Check sheet for the modelled part. Datum: model origin and axes. Units: mm. A direction names the side the tool comes from. Give positions to 0.01 mm unless a question says otherwise; leave off trailing zeros. Write each loop counter-clockwise with the first axis right and the second up, starting at its lowest first coordinate (ties: lowest second). Pieces come first, ordered by that corner, then holes. Notation, with made-up numbers: (68, 9.5) -> (124, 9.5) arc R3 ccw to (124, 13.5) -> close; hole circle Ø3 at (29, 33). An arc over 180 degrees is marked (long way). Use a Markdown table: item, result. Add a question column.
1. Cross-section at C-C (x = -41). Enter the section's corners in (y, z) (1 decimal).
2. Gauge pin test, flat ends, axial feed: P1, Ø1.5, axis at y = -63, z = 8, coming from the -X side; P2, Ø4, axis at x = -23.1, y = 0, coming from the +Z side; P3, Ø8, axis at x = 5.5, y = 16.5, coming from the +Z side. Record the tip position at first contact, or that the pin passes through.
3. Cross-section at A-A (x = 5). Enter the section's corners in (y, z) (1 decimal).
4. Release check for a two-part mould opening along Y. For faces 1 (the cylindrical face through (6.46, -73.07, 1.52)), 2 (the flat face through (5, -64, 3)) record: released by +Y, released by -Y, zero draft, split by the parting line, or undercut.
5. Set-up check for faces 3 (the flat face through (10, -64, 1)), 4 (the flat face through (-35, -53, 0)), 5 (the flat face through (-34, -75.359, 4)), 6 (the cylindrical face through (-12.005, -0.533, 6.535)), 7 (the flat face through (-65.048, -65, 8)): record each of +Z, -Z, +X, -X, +Y, -Y from which the full face is reachable in a straight line by a thin tool's end or side.
6. Cross-section at B-B (y = 0). Enter the section's corners in (x, z).
7. Scan lines: probe 1 along Y at (x, z) = (-33.5, 3) (3 decimals); probe 2 along Y at (x, z) = (5, 1.2) (3 decimals); probe 3 along Y at (x, z) = (-22.5, 8.5) (3 decimals). Record each from-to range of solid material in increasing order. Write a range as [from, to].
8. Cross-section at D-D (y = 30). Enter the section's corners in (x, z).
from build123d import *

# Parameters (mm, degrees)
PAD_DEPTH            = 83.675
POCKET001_DEPTH      = 5
SKETCH003_R          = 1.58
POCKET002_DEPTH      = 9.001
SKETCH006_R          = 1.58
POCKET_DEPTH         = 379.711606
POCKET_DEPTH_BACK    = 388.711606
SKETCH008_R          = 1.58
POCKET004_DEPTH      = 0.001
POCKET004_DEPTH_BACK = 9.001
POCKET005_DEPTH      = 0.001
POCKET005_DEPTH_BACK = 9.001
POCKET006_DEPTH      = 79.208699
POCKET006_DEPTH_BACK = 10.001
POCKET007_DEPTH      = 0.001
POCKET007_DEPTH_BACK = 9.001
POCKET008_DEPTH      = 3


with BuildPart() as part:
    # Sketch → Pad (new body, symmetric)
    with BuildSketch(Plane.XZ):
        Polygon((-6, 9), (-79.207699, 9), (-79.207699, 0), (0, 0), (10, 0), (10, 3), (0, 3), (0, 9), align=None)
    extrude(amount=PAD_DEPTH, both=True)

    # Sketch002 → Pocket001 (cut)
    with BuildSketch(Plane.XY.offset(9)):
        with BuildLine():
            Line((-34.353849, 27.1), (-39.603849, 27.1))
            Line((-39.603849, 27.1), (-44.853849, 27.1))
            ThreePointArc((-44.853849, 27.1), (-67.207699, 0), (-44.853849, -27.1))
            Line((-44.853849, -27.1), (-34.353849, -27.1))
            ThreePointArc((-34.353849, -27.1), (-12, 0), (-34.353849, 27.1))
        make_face()
    extrude(amount=-POCKET001_DEPTH, mode=Mode.SUBTRACT)

    # Sketch003 → Pocket002 (cut, through all)
    with BuildSketch(Plane.XY):
        with Locations((-50.806289, -19.403194)):
            Circle(SKETCH003_R)
        with Locations((-28.40141, -19.403194)):
            Circle(SKETCH003_R)
        with Locations((-28.40141, 19.403194)):
            Circle(SKETCH003_R)
        with Locations((-50.806289, 19.403194)):
            Circle(SKETCH003_R)
        with Locations((-62.008728, 0)):
            Circle(SKETCH003_R)
        with Locations((-56.108728, 0)):
            Circle(SKETCH003_R)
        with Locations((-17.198971, 0)):
            Circle(SKETCH003_R)
        with Locations((-23.098971, 0)):
            Circle(SKETCH003_R)
    extrude(amount=POCKET002_DEPTH, mode=Mode.SUBTRACT)

    # Sketch006 → Pocket (cut, two sides)
    with BuildSketch(Plane.XY) as pocket_sk:
        with Locations((5, 73.675)):
            Circle(SKETCH006_R)
    pocket = extrude(amount=-POCKET_DEPTH, mode=Mode.SUBTRACT) + extrude(pocket_sk.sketch, amount=POCKET_DEPTH_BACK, mode=Mode.SUBTRACT)

    # Mirrored: Pocket across Sketch006 H_Axis
    add(pocket.mirror(Plane.ZX), mode=Mode.SUBTRACT)

    # Sketch008 → Pocket004 (cut, two sides)
    with BuildSketch(Plane.XY) as pocket004_sk:
        with Locations((-70.627699, -68.515)):
            Circle(SKETCH008_R)
        with Locations((-70.627699, -60.515)):
            Circle(SKETCH008_R)
    extrude(amount=-POCKET004_DEPTH, mode=Mode.SUBTRACT)
    extrude(pocket004_sk.sketch, amount=POCKET004_DEPTH_BACK, mode=Mode.SUBTRACT)

    # Sketch005 → Pocket005 (cut, two sides)
    with BuildSketch(Plane.XY) as pocket005_sk:
        with BuildLine():
            ThreePointArc((-5.147488, 84.556872), (-51.101438, 66.874328), (-79.207699, 26.445674))
            Line((-79.207699, 26.445674), (-107.360429, 26.445674))
            Line((-107.360429, 26.445674), (-107.360429, 113.139377))
            Line((-5.147488, 113.139377), (-107.360429, 113.139377))
            Line((-5.147488, 84.556872), (-5.147488, 113.139377))
        make_face()
    extrude(amount=-POCKET005_DEPTH, mode=Mode.SUBTRACT)
    extrude(pocket005_sk.sketch, amount=POCKET005_DEPTH_BACK, mode=Mode.SUBTRACT)

    # Sketch009 → Pocket006 (cut, two sides)
    with BuildSketch(Plane.YZ) as pocket006_sk:
        with BuildLine():
            ThreePointArc((-33.515, 0), (-40.015, 4), (-46.515, 0))
            Line((-40.015, 0), (-46.515, 0))
            Line((-40.015, 0), (-33.515, 0))
        make_face()
    extrude(amount=-POCKET006_DEPTH, mode=Mode.SUBTRACT)
    extrude(pocket006_sk.sketch, amount=POCKET006_DEPTH_BACK, mode=Mode.SUBTRACT)

    # Sketch010 → Pocket007 (cut, two sides)
    with BuildSketch(Plane.XY) as pocket007_sk:
        with BuildLine():
            ThreePointArc((-44.458302, -55.549289), (-54.363008, -65.453995), (-44.458302, -75.358701))
            Line((-44.458302, -75.358701), (-22.419182, -75.358701))
            ThreePointArc((-22.419182, -75.358701), (-12.514476, -65.453995), (-22.419182, -55.549289))
            Line((-22.419182, -55.549289), (-44.458302, -55.549289))
        make_face()
    extrude(amount=-POCKET007_DEPTH, mode=Mode.SUBTRACT)
    extrude(pocket007_sk.sketch, amount=POCKET007_DEPTH_BACK, mode=Mode.SUBTRACT)

    # Sketch007 → Pocket008 (cut)
    with BuildSketch(Plane.XY.offset(9)):
        with BuildLine():
            Line((-79.207699, -64.515), (-79.207699, -68.515))
            Line((-76.207699, -68.515), (-79.207699, -68.515))
            ThreePointArc((-76.207699, -68.515), (-70.627699, -74.095), (-65.047699, -68.515))
            Line((-65.047699, -68.515), (-65.047699, -64.515))
            Line((-65.047699, -60.515), (-65.047699, -64.515))
            ThreePointArc((-65.047699, -60.515), (-70.627699, -54.935), (-76.207699, -60.515))
            Line((-76.207699, -60.515), (-79.207699, -60.515))
            Line((-79.207699, -64.515), (-79.207699, -60.515))
        make_face()
    extrude(amount=-POCKET008_DEPTH, mode=Mode.SUBTRACT)


solid = part.part
Worked answers:
| question | item | result |
|---|---|---|
| 1 | outline | (-83.7, 0) -> (-75.4, 0) -> (-75.4, 9) -> (-83.7, 9) -> close; (-55.5, 0) -> (-46.5, 0) arc R7.3 cw to (-33.5, 0) -> (73.7, 0) -> (73.7, 9) -> (27.1, 9) -> (27.1, 4) -> (-27.1, 4) -> (-27.1, 9) -> (-55.5, 9) -> close |
| 2 | P1 | stops at x = -65.05 |
| 2 | P2 | stops at z = 4 |
| 2 | P3 | stops at z = 3 |
| 3 | outline | (-83.7, 0) -> (-75.3, 0) -> (-75.3, 3) -> (-83.7, 3) -> close; (-72.1, 0) -> (-46.5, 0) arc R7.3 cw to (-43.7, 3) -> (-72.1, 3) -> close; (-36.3, 3) arc R7.3 cw to (-33.5, 0) -> (72.1, 0) -> (72.1, 3) -> close; (75.3, 0) -> (83.7, 0) -> (83.7, 3) -> (75.3, 3) -> close |
| 4 | face 1 | undercut |
| 4 | face 2 | zero draft |
| 5 | face 3 | +Z, -Z, +X, +Y, -Y |
| 5 | face 4 | -Z, +X, -X, +Y, -Y |
| 5 | face 5 | +Z, -Z |
| 5 | face 6 | +Z |
| 5 | face 7 | +Z, -X |
| 6 | outline | (-79.21, 0) -> (-63.59, 0) -> (-63.59, 4) -> (-67.21, 4) -> (-67.21, 9) -> (-79.21, 9) -> close; (-60.43, 0) -> (-57.69, 0) -> (-57.69, 4) -> (-60.43, 4) -> close; (-54.53, 0) -> (-24.68, 0) -> (-24.68, 4) -> (-54.53, 4) -> close; (-21.52, 0) -> (-18.78, 0) -> (-18.78, 4) -> (-21.52, 4) -> close; (-15.62, 0) -> (10, 0) -> (10, 3) -> (0, 3) -> (0, 9) -> (-12, 9) -> (-12, 4) -> (-15.62, 4) -> close |
| 7 | probe 1 | y = [-83.675, -75.359], [-55.549, -43.698], [-36.332, 77.484] |
| 7 | probe 2 | y = [-83.675, -75.255], [-72.095, -45.754], [-34.276, 72.095], [75.255, 83.675] |
| 7 | probe 3 | y = [-83.675, -75.359], [-55.549, -21.666], [21.666, 81.496] |
| 8 | outline | (-77.98, 0) -> (10, 0) -> (10, 3) -> (0, 3) -> (0, 9) -> (-77.98, 9) -> close |
